Source: CAD feature listing. Evaluate the final solid. Frame: model axes, mm. A direction names the side the tool comes from. Round coordinates to 2 decimals unless told otherwise and drop trailing zeros. Loops run counter-clockwise (first coordinate to the right, second up) from the corner with the lowest first, then second, coordinate; pieces in that order, holes last. Notation, with made-up numbers: (36, 73) - (88, 73) arc R38 cw to (88, 111) - close; hole circle Ø4 at (87, -30). An arc over 180 degrees is marked (long way). Write item = value, one per line. Start each with the question number.
from build123d import *

# Parameters (mm, degrees)
SKETCH1_W                  = 100
SKETCH1_H                  = 100
BOSS_EXTRUDE1_DEPTH        = 10
HOLE1_D                    = 62.6
HOLE1_DEPTH                = 8.6
SKETCH4_W                  = 27.8
SKETCH4_H                  = 2.25
SKETCH5_W                  = 1.2
SKETCH5_H                  = 6.35
F_10_CLEARANCE_HOLE1_D     = 5.1
F_10_CLEARANCE_HOLE1_DEPTH = 6
HOLE2_D                    = 52
FILLET1_R                  = 5


with BuildPart() as part:
    # Sketch1 → Boss-Extrude1 (new body)
    with BuildSketch(Plane(origin=(0, 0, 0), x_dir=(-1, 0, 0), z_dir=(0, 0, -1))):
        with Locations((-50, 50)):
            Rectangle(SKETCH1_W, SKETCH1_H)
    extrude(amount=-BOSS_EXTRUDE1_DEPTH)

    # Hole1
    with Locations(Plane.XY.offset(10)):
        with Locations((50, 50)):
            Hole(HOLE1_D / 2, depth=HOLE1_DEPTH)

    # Sketch4 → Revolve1 (revolve)
    with BuildSketch(Plane.XZ.offset(-50)):
        with Locations((63.9, 2.525)):
            Rectangle(SKETCH4_W, SKETCH4_H)
    revolve(axis=Axis((50, 50, 3.65), (0, 0, -1)))

    # Sketch5 → Cut-Revolve1 (revolve, cut)
    with BuildSketch(Plane.XZ.offset(-50), mode=Mode.PRIVATE) as cut_revolve1_sk:
        with Locations((81.9, 6.825)):
            Rectangle(SKETCH5_W, SKETCH5_H)
    revolve(cut_revolve1_sk.sketch.rotate(Axis((50, 50, 10), (0, 0, -1)), 180), axis=Axis((50, 50, 10), (0, 0, -1)), mode=Mode.SUBTRACT)

    # #10 Clearance Hole1
    with Locations(Plane.XY.offset(10)):
        with Locations((80, 80), (80, 20), (20, 20), (20, 80)):
            Hole(F_10_CLEARANCE_HOLE1_D / 2, depth=F_10_CLEARANCE_HOLE1_DEPTH)

    # Hole2 (through all)
    with Locations(Plane.XY.offset(3.65)):
        with Locations((50, 50)):
            Hole(HOLE2_D / 2)

    # Fillet1
    fillet1_edges = [part.edges().sort_by_distance(p)[0] for p in [
        (100, 100, 5),
        (0, 100, 5),
        (0, 0, 5),
        (100, 0, 5),
    ]]
    fillet(fillet1_edges, radius=FILLET1_R)


solid = part.part
(1) Pin query (flat end, axial travel): P1, Ø1.5, axis at x = 79.5, y = 80, coming from the +Z side; P2, Ø2, axis at x = 80.5, y = 42.5, coming from the +Z side; P3, Ø4, axis at x = 79.5, y = 20.5, coming from the +Z side. Return the tip coordinate at first contact, or that it passes through.
(2) Access query for faces 4 (the face through (80, 80, 4)), 5 (the face through (100, 49, 5)). Directions: +Z, -Z, +X, -X, +Y, -Y. A direction counts if a zero-diameter tool reaches every point of the face in a straight line with its end or side. Return the directions, or none.
(3) Cut plane D-D (x = 20). Output: boundary loops of the cut face in (y, z).
(4) Cut plane A-A (y = 50). Output: boundary loops of the cut face in (x, z).
(5) Mould query, pull axis Y, two halves, no side actions, for faces 1 (the face through (22.548, 20.112, 6.958)), 2 (the face through (51, 100, 5)), 3 (the face through (99, 2, 5)). Classes: +Y half, -Y half, draft (parallel to the pull), parting line (faces both ways), or undercut.
(6) Material intervals for line 1 along Y through (x, z) = (50, 3.05); line 2 along Y through (x, z) = (50, 5); line 3 along X through (y, z) = (42, 3), sorted ascending. Write a range as from..to.
(7) Cut plane C-C (z = 7). Output: boundary loops of the cut face in (x, y).
Solution:
q1.P1 = 4
q1.P2 = 3.65
q1.P3 = 10
q2.face_4 = +Z
q2.face_5 = +Z, -Z, +X, +Y, -Y
q3.outline = (0, 0) - (100, 0) - (100, 10) - (82.55, 10) - (82.55, 4) - (77.45, 4) - (77.45, 10) - (62.5, 10) - (62.5, 3.65) - (58.93, 3.65) - (58.93, 1.4) - (41.07, 1.4) - (41.07, 3.65) - (37.5, 3.65) - (37.5, 10) - (22.55, 10) - (22.55, 4) - (17.45, 4) - (17.45, 10) - (0, 10) - close
q4.outline = (0, 0) - (24, 0) - (24, 3.65) - (22.2, 3.65) - (22.2, 1.4) - (18.7, 1.4) - (18.7, 3.65) - (17.5, 3.65) - (17.5, 10) - (0, 10) - close; (76, 0) - (100, 0) - (100, 10) - (82.5, 10) - (82.5, 3.65) - (81.3, 3.65) - (81.3, 1.4) - (77.8, 1.4) - (77.8, 3.65) - (76, 3.65) - close
q5.face_1 = undercut
q5.face_2 = +Y half
q5.face_3 = -Y half
q6.line_1 = 0..18.7, 22.2..24, 76..77.8, 81.3..100
q6.line_2 = 0..17.5, 82.5..100
q6.line_3 = 0..19.74, 23.38..25.26, 74.74..76.62, 80.26..100
q7.outline = (0, 5) arc R5 ccw to (5, 0) - (95, 0) arc R5 ccw to (100, 5) - (100, 95) arc R5 ccw to (95, 100) - (5, 100) arc R5 ccw to (0, 95) - close; hole circle Ø5.1 at (20, 20); hole circle Ø5.1 at (20, 80); hole circle Ø65 at (50, 50); hole circle Ø5.1 at (80, 20); hole circle Ø5.1 at (80, 80)
